Geometry: final body of the model. Coordinates: model frame, mm. A direction names the side the tool comes from. Round coordinates to 2 decimals unless told otherwise and drop trailing zeros. Loops run counter-clockwise (first coordinate to the right, second up) from the corner with the lowest first, then second, coordinate; pieces in that order, holes last. Notation, with made-up numbers: (52.5, 47.25) -> (109.5, 47.25) arc R27 cw to (109.5, 85.25) -> close; hole circle Ø11 at (-38, 26). An arc over 180 degrees is marked (long way). Answer in a Markdown table with one row per item.
```python
from build123d import *

# Parameters (mm, degrees)
F1_DEPTH      = 300
F1_DEPTH_BACK = 300
F2_R          = 255
F3_DEPTH      = 500
F4_R          = 255
F5_DEPTH      = 500


with BuildPart() as f1:
    # F0 (on Front) → F1 (new body, two sides)
    with BuildSketch(Plane.XZ) as f1_sk:
        Polygon((-300, 0), (0, 0), (150, 259.8076211353), (145.6698729811, 262.3076211353), (-2.8867513459, 5), (-300, 5), align=None)
    extrude(amount=F1_DEPTH)
    extrude(f1_sk.sketch, amount=-F1_DEPTH_BACK)

    # F2 (on Top) → F3 (intersect)
    with BuildSketch(Plane.XY):
        Circle(F2_R)
    extrude(amount=F3_DEPTH, mode=Mode.INTERSECT)

    # F4 (on face) → F5 (intersect)
    with BuildSketch(Plane(origin=(0, 0, 0), x_dir=(0, 1, 0), z_dir=(0.8660254038, 0, -0.5))):
        Circle(F4_R)
    extrude(amount=-F5_DEPTH, mode=Mode.INTERSECT)


solid = f1.part
```
Item 1: Pin query (flat end, axial travel): pin 1 Ø12 at (x, y) = (-182.5, -101) entering from +Z; pin 2 Ø2 at (y, z) = (-188, 110.5) entering from +X; pin 3 Ø3 at (y, z) = (-106.5, 88.5) entering from +X. Return the tip coordinate at first contact, or that it passes through.
Answer:
| item | result |
|---|---|
| pin 1 | stops at z = 5 |
| pin 2 | stops at x = 64.37 |
| pin 3 | stops at x = 51.96 |
Item 2: Cut plane A-A (y = 0). Output: boundary loops of the cut face in (x, z), then the cut area to 3 significant figures.
Answer:
| item | result |
|---|---|
| outline | (-255, 0) -> (0, 0) -> (127.5, 220.84) -> (123.17, 223.34) -> (-2.89, 5) -> (-255, 5) -> close |
| area | 2,540 mm² |
Item 3: Cut plane C-C (y = 189). Output: boundary loops of the cut face in (x, z), then the cut area to 3 significant figures.
Answer:
| item | result |
|---|---|
| outline | (-171.18, 0) -> (0, 0) -> (85.59, 148.25) -> (81.26, 150.75) -> (-2.89, 5) -> (-171.18, 5) -> close |
| area | 1,700 mm² |
Item 4: Reachability of faces 1 (the face through (-99, -4, 5)), 2 (the face through (-101, -4, 0)) from +Z, -Z, +X, -X, +Y, -Y: full face, straight path, thin tool, end or side. Return the list, or none.
Answer:
| item | result |
|---|---|
| face 1 | +Z, -X, +Y, -Y |
| face 2 | -Z, +X, -X, +Y, -Y |
Item 5: Line query: probe 1 along Z at (x, y) = (-137, 78); probe 2 along Z at (x, y) = (35.5, -176); probe 3 along X at (y, z) = (-84.5, 75.5). Output: solid intervals per line, ascending. Write a range as [from, to].
Answer:
| item | result |
|---|---|
| probe 1 | z = [0, 5] |
| probe 2 | z = [61.49, 71.49] |
| probe 3 | x = [37.82, 43.59] |
Item 6: Cut plane B-B (x = -148). Output: boundary loops of the cut face in (y, z), then the cut area to 3 significant figures.
Answer:
| item | result |
|---|---|
| outline | (-207.66, 0) -> (207.66, 0) -> (207.66, 5) -> (-207.66, 5) -> close |
| area | 2,080 mm² |
